Input: part model. Units: mm. Frame: model coordinates. A direction names the side the tool comes from. Coordinates: 2 decimals unless noted, no trailing zeros. Write each loop counter-clockwise with the first axis right and the second up, starting at its lowest first coordinate (ties: lowest second). Pieces come first, ordered by that corner, then holes. Notation, with made-up numbers: (63.25, 2.5) - (113.25, 2.5) arc R30 cw to (113.25, 35.5) - close; hole circle Ø4 at (14.25, -33). An arc over 180 degrees is marked (long way). Use a Markdown table: item, result. Add a question column.
Q1. Pin query (flat end, axial travel): P1, Ø20.5, axis at y = 0, z = 0, coming from the +X side; P2, Ø8, axis at x = 18, z = -12, coming from the -Y side; P3, Ø5, axis at x = -10, y = -13, coming from the -Z side; P4, Ø4, axis at y = -4, z = 8.5, coming from the +X side. Return the tip coordinate at first contact, or that it passes through.
Q2. Section query A-A (y = 0). Return the cut outline in (x, z) (3 decimals), then the cut area to 3 significant figures.
Q3. Section query D-D (z = 10.5). Return the cut outline in (x, y) (3 decimals).
Q4. Material intervals for probe 1 along Z at (x, y) = (28, 0); probe 2 along Z at (x, y) = (27, -3), sorted ascending. Write a range as from..to.
Q5. Section query B-B (x = 0). Return the cut outline in (y, z) (3 decimals).
Q6. Set-up query: faces 1 (the face through (35.22, 5.72, -18.17)), 2 (the face through (-19.03, 0.84, -0.36)). Return all of +Z, -Z, +X, -X, +Y, -Y with unobstructed straight access to the full face (end or side cutting, diameter ignored); none if empty.
Q7. Section query C-C (z = 20). Return the cut outline in (x, y) (3 decimals).
from build123d import *

# Parameters (mm, degrees)
SKETCH1_R           = 19.05
SKETCH1_R_2         = 12.7
BOSS_EXTRUDE1_DEPTH = 50.8
SKETCH2_R           = 22.225
SKETCH2_R_2         = 19.05
BOSS_EXTRUDE2_DEPTH = 25.4
CUT_EXTRUDE1_START  = -50.8
SKETCH3_R           = 19.05
CUT_EXTRUDE1_DEPTH  = 50.8
CUT_EXTRUDE2_START  = -50.8
SKETCH4_R           = 12.7
CUT_EXTRUDE2_DEPTH  = 50.8


with BuildPart() as part:
    # Sketch1 → Boss-Extrude1 (new body)
    with BuildSketch(Plane.YZ):
        with Locations(Location((0, 0, 0), (0, 0, 270))):
            Circle(SKETCH1_R)
        with Locations(Location((0, 0, 0), (0, 0, 270))):
            Circle(SKETCH1_R_2, mode=Mode.SUBTRACT)
    extrude(amount=BOSS_EXTRUDE1_DEPTH)

    # Sketch2 → Boss-Extrude2 (add, symmetric)
    with BuildSketch(Plane(origin=(0, 0, 0), x_dir=(0, 1, 0), z_dir=(0, 0, 1))):
        with Locations(Location((0, 0, 0), (0, 0, 270))):
            Circle(SKETCH2_R)
        with Locations(Location((0, 0, 0), (0, 0, 270))):
            Circle(SKETCH2_R_2, mode=Mode.SUBTRACT)
    extrude(amount=BOSS_EXTRUDE2_DEPTH, both=True)

    # Sketch3 → Cut-Extrude1 (cut)
    with BuildSketch(Plane.XY.offset(25.4).offset(CUT_EXTRUDE1_START)):
        Circle(SKETCH3_R)
    extrude(amount=CUT_EXTRUDE1_DEPTH, mode=Mode.SUBTRACT)

    # Sketch4 → Cut-Extrude2 (cut)
    with BuildSketch(Plane.YZ.offset(50.8).offset(CUT_EXTRUDE2_START)):
        with Locations(Location((0, 0, 0), (0, 0, 270))):
            Circle(SKETCH4_R)
    extrude(amount=CUT_EXTRUDE2_DEPTH, mode=Mode.SUBTRACT)


solid = part.part
Values follow:
| question | item | result |
|---|---|---|
| 1 | P1 | x = -16.06 |
| 1 | P2 | y = -17.29 |
| 1 | P3 | through |
| 1 | P4 | x = -18.08 |
| 2 | outline | (-22.225, -25.4) - (-19.05, -25.4) - (-19.05, 25.4) - (-22.225, 25.4) - close; (19.05, -25.4) - (22.225, -25.4) - (22.225, -19.05) - (50.8, -19.05) - (50.8, -12.7) - (19.05, -12.7) - close; (19.05, 12.7) - (50.8, 12.7) - (50.8, 19.05) - (22.225, 19.05) - (22.225, 25.4) - (19.05, 25.4) - close |
| 2 | area | 605 mm2 |
| 3 | outline | (15.534, -15.895) - (50.8, -15.895) - (50.8, -7.144) - (17.66, -7.144) arc R19.05 cw (long way) to (17.66, 7.144) - (50.8, 7.144) - (50.8, 15.895) - (15.534, 15.895) arc R22.225 ccw (long way) to start |
| 4 | probe 1 | -19.05..-12.7, 12.7..19.05 |
| 4 | probe 2 | -18.81..-12.34, 12.34..18.81 |
| 5 | outline | (-22.225, -25.4) - (-19.05, -25.4) - (-19.05, 25.4) - (-22.225, 25.4) - close; (19.05, -25.4) - (22.225, -25.4) - (22.225, 25.4) - (19.05, 25.4) - close |
| 6 | face 1 | +X |
| 6 | face 2 | +Z, -Z |
| 7 | outline | circle Ø44.45 at (0, 0); hole circle Ø38.1 at (0, 0) |
